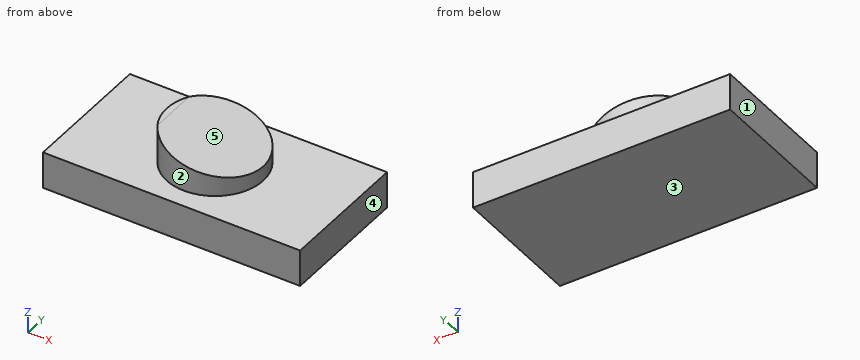
from build123d import *

# Parameters (mm, degrees)
F0_W     = 177.951604
F0_H     = 92.412182
F0_R     = 33.419382
F1_DEPTH = 25.4
F2_DEPTH = 50.8
F4_DEPTH = 38.1


with BuildPart() as f1:
    # F0 (on Top) → F1 (new body)
    with BuildSketch(Plane.XY):
        Rectangle(F0_W, F0_H)
        Circle(F0_R, mode=Mode.SUBTRACT)
        Circle(F0_R)
    extrude(amount=F1_DEPTH)

    # F0 (on Top) → F2 (join)
    with BuildSketch(Plane.XY):
        Circle(F0_R)
    extrude(amount=F2_DEPTH)

    # F3 (on Front) → F4 (cut, symmetric)
    with BuildSketch(Plane.XZ):
        Polygon((44.763692, 56.282684), (-43.013971, 54.241341), (44.763692, 32.953072), align=None)
    extrude(amount=F4_DEPTH, both=True, mode=Mode.SUBTRACT)


solid = f1.part
The listing builds one solid part. Answer for the finished solid, in the listing's coordinates (mm). Face numbers are marked on the shaded views. A direction names the side the tool comes from. Round coordinates to 2 decimals unless told otherwise and drop trailing zeros. Write each loop counter-clockwise with the first axis right and the second up, starting at its lowest first coordinate (ties: lowest second). Pieces come first, ordered by that corner, then holes. Notation, with made-up numbers: (29, 84) - (85, 84) arc R30 ccw to (85, 122) - close; hole circle Ø10 at (56, 38). An arc over 180 degrees is marked (long way). Use a Markdown table: item, result. Add a question column.
1. The part is cut by section C-C (z = 33.5). Write down the section's boundary in (x, y).
2. For a pull along Z with two mould halves and no side action, classify the marked faces 3, 4 and 5 as +Z half, -Z half, draft (parallel to the pull), parting line (faces both ways), or undercut.
3. A tool of negligible diameter and unlimited length cuts with its end or side. For the marked faces 1 and 2, from which of +Z, -Z, +X, -X, +Y, -Y can it reach the whole face along a straight path? Write none if from no direction.
4. The part is cut by section D-D (y = 12). Write down the section's boundary in (x, z).
5. Consider line 1 (Z direction, x = 46.5, y = 16.5); line 2 (Z direction, x = -6, y = 13); line 3 (Y direction, x = -29.5, z = 42). Determine where each line is inside the solid, lowest interval first.
6. The part is cut by section A-A (x = 13.5). Write down the section's boundary in (y, z), and give its area (3 significant figures).
7. The part is cut by section B-B (y = 0). Write down the section's boundary in (x, z).
8. Flat-ended cylindrical pins translate along their axes: P1, Ø5, axis at x = -5.5, y = -24, coming from the +Z side; P2, Ø8, axis at x = -67.5, y = -22, coming from the +Z side; P3, Ø4, axis at y = -19, z = 34.5, coming from the -X side. Find the tip coordinate at first contact, or state that the pin passes through.
Reported:
| question | item | result |
|---|---|---|
| 1 | outline | circle Ø66.84 at (0, 0) |
| 2 | face 3 | -Z half |
| 2 | face 4 | draft |
| 2 | face 5 | +Z half |
| 3 | face 1 | +Z, -Z, -X, +Y, -Y |
| 3 | face 2 | +Z |
| 4 | outline | (-88.98, 0) - (88.98, 0) - (88.98, 25.4) - (31.19, 25.4) - (31.19, 36.24) - (-28.82, 50.8) - (-31.19, 50.8) - (-31.19, 25.4) - (-88.98, 25.4) - close |
| 5 | line 1 | 0 to 25.4 |
| 5 | line 2 | 0 to 45.26 |
| 5 | line 3 | -15.7 to 15.7 |
| 6 | outline | (-46.21, 0) - (46.21, 0) - (46.21, 25.4) - (30.57, 25.4) - (30.57, 40.54) - (-30.57, 40.54) - (-30.57, 25.4) - (-46.21, 25.4) - close |
| 6 | area | 3,270 mm^2 |
| 7 | outline | (-88.98, 0) - (88.98, 0) - (88.98, 25.4) - (33.42, 25.4) - (33.42, 35.7) - (-28.82, 50.8) - (-33.42, 50.8) - (-33.42, 25.4) - (-88.98, 25.4) - close |
| 8 | P1 | z = 45.75 |
| 8 | P2 | z = 25.4 |
| 8 | P3 | x = -28.77 |
